Build history of the part. All positions in model axes, mm. A direction names the side the tool comes from. Coordinates: 2 decimals unless noted, no trailing zeros. Loops run counter-clockwise (first coordinate to the right, second up) from the corner with the lowest first, then second, coordinate; pieces in that order, holes last. Notation, with made-up numbers: M 7.25,11.25 L 66.25,11.25 A24 ccw 66.25,30.25 Z; hole C 78.25,11 d7. An arc over 180 degrees is marked long. Write each question's results on one line, items separated by ' | '. Start each with the question number.
from build123d import *

# Parameters (mm, degrees)
SKETCH1_W                                            = 170
SKETCH1_H                                            = 75
BOSS_EXTRUDE1_DEPTH                                  = 15
SKETCH2_W                                            = 130
SKETCH2_H                                            = 20
CUT_EXTRUDE1_DEPTH                                   = 95.107651124
CBORE_FOR_M3_HEXAGON_SOCKET_HEAD_CAP_SCR_D           = 3.2
CBORE_FOR_M3_HEXAGON_SOCKET_HEAD_CAP_SCR_CBORE_D     = 6
CBORE_FOR_M3_HEXAGON_SOCKET_HEAD_CAP_SCR_CBORE_DEPTH = 3.4
MIRROR2_AT_THE_SECOND_PLANE_COPY_1_D                 = 3.2
MIRROR2_AT_THE_SECOND_PLANE_COPY_1_CBORE_D           = 6
MIRROR2_AT_THE_SECOND_PLANE_COPY_1_CBORE_DEPTH       = 3.4
FILLET1_R                                            = 3
SKETCH9_W                                            = 170
SKETCH9_H                                            = 45
BOSS_EXTRUDE3_DEPTH                                  = 30
SKETCH8_W                                            = 148
SKETCH8_H                                            = 25
CUT_EXTRUDE2_DEPTH                                   = 104.22911411
SKETCH10_W                                           = 162
SKETCH10_H                                           = 37
CUT_EXTRUDE3_DEPTH                                   = 25
FILLET2_R                                            = 3


with BuildPart() as part:
    # Sketch1 → Boss-Extrude1 (new body)
    with BuildSketch(Plane.XY):
        Rectangle(SKETCH1_W, SKETCH1_H)
    extrude(amount=BOSS_EXTRUDE1_DEPTH)

    # Sketch2 → Cut-Extrude1 (cut, through all)
    with BuildSketch(Plane.XY.offset(15)):
        with Locations((0, -27.5)):
            Rectangle(SKETCH2_W, SKETCH2_H)
    cut_extrude1 = extrude(amount=-CUT_EXTRUDE1_DEPTH, mode=Mode.SUBTRACT)

    # Mirror1: Cut-Extrude1 across plane
    add(cut_extrude1.mirror(Plane.ZX), mode=Mode.SUBTRACT)

    # CBORE for M3 Hexagon socket head cap screws1 (through all)
    with Locations(Plane.XY.offset(15)):
        with Locations((-75, 27.5)):
            cbore_for_m3_hexagon_socket_head_cap_scr = CounterBoreHole(CBORE_FOR_M3_HEXAGON_SOCKET_HEAD_CAP_SCR_D / 2, CBORE_FOR_M3_HEXAGON_SOCKET_HEAD_CAP_SCR_CBORE_D / 2, CBORE_FOR_M3_HEXAGON_SOCKET_HEAD_CAP_SCR_CBORE_DEPTH)

    # Mirror2: CBORE for M3 Hexagon socket head cap screws1 across plane
    add(cbore_for_m3_hexagon_socket_head_cap_scr.mirror(Plane(origin=(0, 0, 0), x_dir=(0, 0, 1), z_dir=(1, 0, 0))), mode=Mode.SUBTRACT)

    # Mirror2 at the second plane: CBORE for M3 Hexagon socket head cap screws1 across plane
    add(cbore_for_m3_hexagon_socket_head_cap_scr.mirror(Plane.ZX), mode=Mode.SUBTRACT)

    # Mirror2 at the second plane copy 1 (through all)
    with Locations(Plane(origin=(0, 0, 15), x_dir=(-1, 0, 0), z_dir=(0, 0, 1))):
        with Locations((-75, 27.5)):
            CounterBoreHole(MIRROR2_AT_THE_SECOND_PLANE_COPY_1_D / 2, MIRROR2_AT_THE_SECOND_PLANE_COPY_1_CBORE_D / 2, MIRROR2_AT_THE_SECOND_PLANE_COPY_1_CBORE_DEPTH)

    # Fillet1
    fillet1_edges = [part.edges().sort_by_distance(p)[0] for p in [
        (-65, -17.5, 7.5),
        (65, -17.5, 7.5),
        (-65, 17.5, 7.5),
        (65, 17.5, 7.5),
    ]]
    fillet(fillet1_edges, radius=FILLET1_R)

    # Sketch9 → Boss-Extrude3 (add)
    with BuildSketch(Plane.XY.offset(15)):
        Rectangle(SKETCH9_W, SKETCH9_H)
    extrude(amount=BOSS_EXTRUDE3_DEPTH)

    # Sketch8 → Cut-Extrude2 (cut, through all)
    with BuildSketch(Plane(origin=(0, 0, 0), x_dir=(-1, 0, 0), z_dir=(0, 0, -1))):
        Rectangle(SKETCH8_W, SKETCH8_H)
    extrude(amount=-CUT_EXTRUDE2_DEPTH, mode=Mode.SUBTRACT)

    # Sketch10 → Cut-Extrude3 (cut)
    with BuildSketch(Plane.XY.offset(45)):
        Rectangle(SKETCH10_W, SKETCH10_H)
    extrude(amount=-CUT_EXTRUDE3_DEPTH, mode=Mode.SUBTRACT)

    # Fillet2
    fillet2_edges = [part.edges().sort_by_distance(p)[0] for p in [
        (-74, -12.5, 10),
        (74, -12.5, 10),
        (-74, 12.5, 10),
        (74, 12.5, 10),
        (-81, -18.5, 32.5),
        (-81, 18.5, 32.5),
        (81, 18.5, 32.5),
        (81, -18.5, 32.5),
    ]]
    fillet(fillet2_edges, radius=FILLET2_R)


solid = part.part
1. Band-saw the part on A-A, the plane x = 30.5. List the corners of the cut face in (y, z), plus the area to 3 significant figures.
2. Band-saw the part on D-D, the plane z = 27.5. List the corners of the cut face in (x, y).
3. Which spindle directions (+Z, -Z, +X, -X, +Y, -Y) get a long thin tool onto all of the face, cutting with end or side? Do faces 1 (the cylindrical face through (64.1, -18.36, 7.4)), 2 (the flat face through (0, -14, 20)), 3 (the cylindrical face through (-73.14, -11.6, 10.14)), 4 (the flat face through (75, 32, 15)), 5 (the flat face through (-1, 20, 15)). Say none if no direction does.
4. Band-saw the part on C-C, the plane z = 10. List the corners of the cut face in (x, y), plus the area to 3 significant figures.
5. Mould opens along X. For faces 6 (the cylindrical face through (80.1, -17.64, 32.33)), 7 (the flat face through (75, -32, 15)), 8 (the flat face through (-85, -1, 17)) say: +X half, -X half, draft (parallel to the pull), parting line (faces both ways), or undercut.
6. Band-saw the part on B-B, the plane y = 32.5. List the corners of the cut face in (x, z), plus the area to 3 significant figures.
7. Pin check, flat tips, straight feed: pin 1 (20 mm diameter, centred on x = 27, z = 37, fed in from -Y); pin 2 (3 mm diameter, centred on x = 73.5, y = 28, fed in from +Z); pin 3 (1 mm diameter, centred on x = -13.5, y = -16, fed in from +Z); pin 4 (4 mm diameter, centred on x = 75, y = 27.5, fed in from -Z). Stop position of each tip, or through.
8. Wall check: line 1 along Y through (x, z) = (75, 13.9); line 2 along Y through (x, z) = (75, 2.5); line 3 along Y through (x, z) = (-52.5, 25). Give the ranges that are in metal, low to high.
Checked values:
1) outline: M -22.5,15 L -17.5,15 L -17.5,0 L -12.5,0 L -12.5,20 L -18.5,20 L -18.5,45 L -22.5,45 Z; M 12.5,0 L 17.5,0 L 17.5,15 L 22.5,15 L 22.5,45 L 18.5,45 L 18.5,20 L 12.5,20 Z | area: 450 mm²
2) outline: M -85,-22.5 L 85,-22.5 L 85,22.5 L -85,22.5 Z; hole M -81,-15.5 A3 ccw -78,-18.5 L 78,-18.5 A3 ccw 81,-15.5 L 81,15.5 A3 ccw 78,18.5 L -78,18.5 A3 ccw -81,15.5 Z
3) face 1: -Z, -Y | face 2: +Z | face 3: +Z, -Z | face 4: +Z, +X, -X, +Y | face 5: -Z, +Y
4) outline: M -85,-37.5 L -65,-37.5 L -65,-20.5 A3 cw -62,-17.5 L 62,-17.5 A3 cw 65,-20.5 L 65,-37.5 L 85,-37.5 L 85,37.5 L 65,37.5 L 65,20.5 A3 cw 62,17.5 L -62,17.5 A3 cw -65,20.5 L -65,37.5 L -85,37.5 Z; hole C -75,-27.5 d3.2; hole C -75,27.5 d3.2; hole M -74,-9.5 A3 ccw -71,-12.5 L 71,-12.5 A3 ccw 74,-9.5 L 74,9.5 A3 ccw 71,12.5 L -71,12.5 A3 ccw -74,9.5 Z; hole C 75,-27.5 d3.2; hole C 75,27.5 d3.2 | area: 3,830 mm²
5) face 6: undercut | face 7: draft | face 8: -X half
6) outline: M -85,0 L -65,0 L -65,15 L -85,15 Z; M 65,0 L 85,0 L 85,15 L 65,15 Z | area: 600 mm²
7) pin 1: y = -22.5 | pin 2: z = 15 | pin 3: z = 20 | pin 4: z = 0
8) line 1: -37.5 to -30.5, -24.5 to 24.5, 30.5 to 37.5 | line 2: -37.5 to -29.1, -25.9 to 25.9, 29.1 to 37.5 | line 3: -22.5 to -18.5, 18.5 to 22.5
